Can you work these out from the model? Positions are in its coordinate system, mm. Round coordinates to 2 decimals unless told otherwise and drop trailing zeros. Order: outer loops, then holes, each group sorted by start corner. A loop starts at its lowest first (then second) coordinate and runs counter-clockwise, first axis right, second up. Notation, with made-up numbers: (13, -7.5) -> (72, -7.5) arc R17 ccw to (72, 0.5) -> close; hole circle Ø9 at (76.25, 6). An arc over 180 degrees is marked (long way). One line per item, written item: value.
```python
from build123d import *

# Parameters (mm, degrees)
SKETCH1_R                                       = 75
BOSS_EXTRUDE1_DEPTH                             = 10
CSK_FOR_M3_FLAT_HEAD_MACHINE_SCREW1_D           = 3.4
CSK_FOR_M3_FLAT_HEAD_MACHINE_SCREW1_CSINK_D     = 6.3
CSK_FOR_M3_FLAT_HEAD_MACHINE_SCREW1_CSINK_ANGLE = 90
CIRPATTERN1_COUNT                               = 4
SKETCH8_R                                       = 7.5
CUT_EXTRUDE1_DEPTH                              = 107.536378763
CSK_FOR_M3_FLAT_HEAD_MACHINE_SCREW2_D           = 3.4
CSK_FOR_M3_FLAT_HEAD_MACHINE_SCREW2_CSINK_D     = 6.3
CSK_FOR_M3_FLAT_HEAD_MACHINE_SCREW2_CSINK_ANGLE = 90
FILLET1_R                                       = 1


with BuildPart() as part:
    # Sketch1 → Boss-Extrude1 (new body)
    with BuildSketch(Plane(origin=(0, 0, 0), x_dir=(1, 0, 0), z_dir=(0, 1, 0))):
        with Locations(Location((0, 0, 0), (0, 0, 270))):
            Circle(SKETCH1_R)
    extrude(amount=BOSS_EXTRUDE1_DEPTH)

    # CSK for M3 Flat Head Machine Screw1 (through all)
    with Locations(Plane(origin=(0, 10, 0), x_dir=(1, 0, 0), z_dir=(0, 1, 0))):
        with Locations((0, 70)):
            csk_for_m3_flat_head_machine_screw1 = CounterSinkHole(CSK_FOR_M3_FLAT_HEAD_MACHINE_SCREW1_D / 2, CSK_FOR_M3_FLAT_HEAD_MACHINE_SCREW1_CSINK_D / 2, counter_sink_angle=CSK_FOR_M3_FLAT_HEAD_MACHINE_SCREW1_CSINK_ANGLE)

    # CirPattern1: CSK for M3 Flat Head Machine Screw1 ×4 about axis
    cirpattern1_axis = Axis((0, 0, 0), (0, 1, 0))
    for i in range(1, CIRPATTERN1_COUNT):
        add(csk_for_m3_flat_head_machine_screw1.rotate(cirpattern1_axis, i * 360 / CIRPATTERN1_COUNT), mode=Mode.SUBTRACT)

    # Sketch8 → Cut-Extrude1 (cut, through all)
    with BuildSketch(Plane(origin=(0, 10, 0), x_dir=(1, 0, 0), z_dir=(0, 1, 0))):
        with Locations(Location((0, 0, 0), (0, 0, 270))):
            Circle(SKETCH8_R)
    extrude(amount=-CUT_EXTRUDE1_DEPTH, mode=Mode.SUBTRACT)

    # CSK for M3 Flat Head Machine Screw2 (through all)
    with Locations(Plane(origin=(0, 10, 0), x_dir=(1, 0, 0), z_dir=(0, 1, 0))):
        with Locations((22.5, 22.5), (22.5, -22.5), (-22.5, -22.5), (-22.5, 22.5)):
            CounterSinkHole(CSK_FOR_M3_FLAT_HEAD_MACHINE_SCREW2_D / 2, CSK_FOR_M3_FLAT_HEAD_MACHINE_SCREW2_CSINK_D / 2, counter_sink_angle=CSK_FOR_M3_FLAT_HEAD_MACHINE_SCREW2_CSINK_ANGLE)

    # Fillet1
    fillet1_edges = [part.edges().sort_by_distance(p)[0] for p in [
        (0, 10, -75),
    ]]
    fillet(fillet1_edges, radius=FILLET1_R)


solid = part.part
```
Q1. I want a section at A-A on z = 0. List the corners of the cut face in (x, y) for me, plus the area to 3 significant figures.
Answers below:
outline: (-75, 0) -> (-71.7, 0) -> (-71.7, 8.55) -> (-73.15, 10) -> (-74, 10) arc R1 ccw to (-75, 9) -> close; (-68.3, 0) -> (-7.5, 0) -> (-7.5, 10) -> (-66.85, 10) -> (-68.3, 8.55) -> close; (7.5, 0) -> (68.3, 0) -> (68.3, 8.55) -> (66.85, 10) -> (7.5, 10) -> close; (71.7, 0) -> (75, 0) -> (75, 9) arc R1 ccw to (74, 10) -> (73.15, 10) -> (71.7, 8.55) -> close
area: 1,280 mm^2
Q2. We'd pull the mould along X, two halves only. Please class faces 1 (the face through (-45.636, 4.437, -59.517)), 2 (the face through (-0.37, 4.22, 68.34)), 3 (the face through (-16, 0, -1)): released by +X, released by -X, zero draft, split by the parting line, or undercut.
Answers below:
face 1: split by the parting line
face 2: undercut
face 3: zero draft
Q3. Will these pins go through, and if not, where does the flat tip stop? pin 1 Ø1 at (x, y) = (44, 4) entering from +Z; pin 2 Ø4 at (y, z) = (8.5, 33) entering from -X; pin 3 Ø4 at (x, z) = (22.5, -22.5) entering from +Y; pin 4 Ø2.5 at (x, z) = (0, -70) entering from +Y.
Answers below:
pin 1: z = 61.1
pin 2: x = -68.29
pin 3: y = 8.85
pin 4: through
Q4. Please list where these lines run through material, in increasing order: line 1 along X through (y, z) = (4.75, 0); line 2 along X through (y, z) = (4.5, -22.5); line 3 along X through (y, z) = (1.75, -24).
Answers below:
line 1: -75 to -71.7, -68.3 to -7.5, 7.5 to 68.3, 71.7 to 75
line 2: -71.55 to -24.2, -20.8 to 20.8, 24.2 to 71.55
line 3: -71.06 to -23.3, -21.7 to 21.7, 23.3 to 71.06
Q5. I want a section at B-B on x = 0. List the corners of the cut face in (y, z) for me.
Answers below:
outline: (0, -75) -> (9, -75) arc R1 ccw to (10, -74) -> (10, -73.15) -> (8.55, -71.7) -> (0, -71.7) -> close; (0, -68.3) -> (8.55, -68.3) -> (10, -66.85) -> (10, -7.5) -> (0, -7.5) -> close; (0, 7.5) -> (10, 7.5) -> (10, 66.85) -> (8.55, 68.3) -> (0, 68.3) -> close; (0, 71.7) -> (8.55, 71.7) -> (10, 73.15) -> (10, 74) arc R1 ccw to (9, 75) -> (0, 75) -> close
Q6. I want a section at C-C on y = 2.5. Give the number of separate pieces and of enclosed holes in the cut face, plus the area to 3 significant figures.
Answers below:
separate pieces: 1
enclosed holes: 9
area: 17,400 mm^2
